Autodesk Inventor part; units mm, degrees
ref_plane "Work Plane1" through (0, -6.35, 0) normal (0, 1, 0) x (-1, 0, 0)
ref_plane "YZ Plane" through (0, 0, 0) normal (1, 0, 0) x (0, 1, 0)
ref_plane "XY Plane" through (0, 0, 0) normal (0, 0, 1) x (1, 0, 0)
sketch "Sketch3" plane through (0, 0, 0) normal (0, 0, 1) x (1, 0, 0)
  circle A0 centre (0, 0) radius 6.35
  dimension "d0" = 12.7
extrude "Extrusion1" add sketch "Sketch3" along normal mid plane 146.05
sketch "Sketch4" plane through (0, 0, 73.025) normal (0, 0, 1) x (1, 0, 0)
  point P0 (0, 0)
  point P1 (-0.1209, -0.1497)
hole "Hole1" at (-0.1209, -0.1497, 73.025) direction (0, 0, -1) diameter 3.9624 depth 25.4 tip angle 118
mirror "Mirror1" about plane through (0, 0, 0) normal (0, 0, 1) of "Hole1"
ref_plane "Work Plane1" through (0, -6.35, 0) normal (0, 1, 0) x (-1, 0, 0)
sketch "Sketch5" plane through (0, -6.35, 0) normal (0, 1, 0) x (-1, 0, 0)
  line L0 (0, 34.925) -> (0, 12.7) construction
  line L1 (-1.6002, 34.925) -> (-1.6002, 12.7)
  line L2 (1.6002, 12.7) -> (1.6002, 34.925)
  arc A0 (1.6002, 34.925) -> (-1.6002, 34.925) centre (0, 34.925) ccw
  arc A1 (-1.6002, 12.7) -> (1.6002, 12.7) centre (0, 12.7) ccw
  point P0 (0, 0)
  point P1 (0, 23.8125)
  dimension "d10" = 3.2004
  dimension "d11" = 23.8125
  dimension "d12" = 22.225
extrude "Extrusion2" cut sketch "Sketch5" along normal blind 1.6002
properties part number "1886K21_Rotary Shaft _Short"
CAD build for the part. Positions are in the model's coordinates, mm. A direction names the side the tool comes from. Give positions to 0.01 mm unless a question says otherwise; leave off trailing zeros. Loops run counter-clockwise (first coordinate to the right, second up) from the corner with the lowest first, then second, coordinate; pieces in that order, holes last. Notation, with made-up numbers: M 60.25,25 L 117.25,25 A29 ccw 117.25,64 Z; hole C 33,65.5 d8. An arc over 180 degrees is marked long. Answer in a Markdown table with one row per item. Add a question column.
Item 1: Probe probe 1 along X at (y, z) = (-1, 47.5); probe 2 along Y at (x, z) = (-1, -64); probe 3 along Y at (x, z) = (0.25, 12). List the from-to ranges inside material, lowest first.
Item 2: Band-saw the part on C-C on x = -4. Give the cut face in (y, z) (3 decimals).
Item 3: Band-saw the part on D-D on z = 62. Give the cut face in (x, y), then the cut area to 3 significant figures.
Item 4: Band-saw the part on A-A on z = -3. Give the cut face in (x, y), then the cut area to 3 significant figures.
Item 5: Band-saw the part on B-B on y = -3.5. Give the cut face in (x, z) (3 decimals).
Item 6: Tool access for faces 4 (the face through (0, -4.75, 24)), 5 (the face through (-2.085, 0.108, 60.147)), 6 (the face through (1, 2, 73.025)), 7 (the face through (1.22, 1.31, -60.15)): list every direction of +Z, -Z, +X, -X, +Y, -Y with a clear straight run to the whole face (end or side of a thin tool).
Item 7: Drop flat-ended pins along their axis: P1, Ø1, axis at x = 3.5, z = -16, coming from the -Y side; P2, Ø1.1, axis at y = -6, z = 26, coming from the -X side; P3, Ø5, axis at y = -4, z = -53, coming from the -X side. Give the stop position or say it passes through.
Item 8: Mould opens along X. For faces 1 (the face through (1, 2, -73.025)), 2 (the face through (-0.426, -0.308, 46.641)), 3 (the face through (-1.38, 6.2, -1.02)) say: +X half, -X half, draft (parallel to the pull), parting line (faces both ways), or undercut.
Reply:
| question | item | result |
|---|---|---|
| 1 | probe 1 | x = -6.27 to -1.68, 1.44 to 6.27 |
| 1 | probe 2 | y = -6.27 to -1.93, 1.63 to 6.27 |
| 1 | probe 3 | y = -4.75 to 6.35 |
| 2 | outline | M -4.932,-73.025 L 4.932,-73.025 L 4.932,73.025 L -4.932,73.025 Z |
| 3 | outline | C 0,0 d12.7; hole C -0.12,-0.15 d3.96 |
| 3 | area | 114 mm^2 |
| 4 | outline | C 0,0 d12.7 |
| 4 | area | 127 mm^2 |
| 5 | outline | M -5.298,-73.025 L 5.298,-73.025 L 5.298,73.025 L -5.298,73.025 Z |
| 6 | face 4 | -Y |
| 6 | face 5 | +Z |
| 6 | face 6 | +Z, +X, -X, +Y, -Y |
| 6 | face 7 | -Z |
| 7 | P1 | stops at y = -5.6 |
| 7 | P2 | stops at x = -3.26 |
| 7 | P3 | stops at x = -6.17 |
| 8 | face 1 | draft |
| 8 | face 2 | undercut |
| 8 | face 3 | parting line |
